Read the model definition and answer for the solid it produces. Units are mm, in the model's axes. A direction names the side the tool comes from. Coordinates: 2 decimals unless noted, no trailing zeros. Write each loop counter-clockwise with the first axis right and the second up, starting at its lowest first coordinate (ties: lowest second). Pieces come first, ordered by that corner, then holes. Notation, with made-up numbers: (20, -12) - (52, -12) arc R9 cw to (52, -3) - close; hole circle Ø6 at (-20.5, 27.5). An arc over 180 degrees is marked (long way). Return JSON: item names as keys, results as strings.
```python
from build123d import *

# Parameters (mm, degrees)
SKETCH1_R           = 15
BOSS_EXTRUDE1_DEPTH = 23.5
SKETCH2_R           = 1.65
CUT_EXTRUDE1_DEPTH  = 10


with BuildPart() as part:
    # Sketch1 → Boss-Extrude1 (new, symmetric)
    with BuildSketch(Plane.XY):
        Circle(SKETCH1_R)
    extrude(amount=BOSS_EXTRUDE1_DEPTH, both=True)

    # Sketch2 → Cut-Extrude1 (cut)
    with BuildSketch(Plane(origin=(0, 0, -23.5), x_dir=(-1, 0, 0), z_dir=(0, 0, -1))):
        with Locations((8, 8)):
            Circle(SKETCH2_R)
        with Locations((8, -8)):
            Circle(SKETCH2_R)
        with Locations((-8, -8)):
            Circle(SKETCH2_R)
        with Locations((-8, 8)):
            Circle(SKETCH2_R)
    extrude(amount=-CUT_EXTRUDE1_DEPTH, mode=Mode.SUBTRACT)


solid = part.part
```
(1) Which of the six approach directions +Z, -Z, +X, -X, +Y, -Y give full straight-line access (tool end or side, diameter ignored) to faces 4 (the face through (0, 0, -23.5)), 5 (the face through (9.65, -7.93, -18.57))?
Answer:
{"face 4": "-Z, +X, -X, +Y, -Y", "face 5": "-Z"}
(2) Determine the mould class of faces 1 (the face through (-14.985, 0.66, 0.329)), 2 (the face through (0, 0, 23.5)), 3 (the face through (-6.784, 9.115, -18.57)) for opening direction Y: +Y half, -Y half, draft (parallel to the pull), parting line (faces both ways), or undercut.
Answer:
{"face 1": "parting line", "face 2": "draft", "face 3": "undercut"}
(3) Straight lines are drawn through the part: line 1 (Y direction, x = 8, z = -19); line 2 (Z direction, x = -8.5, y = 9.5); line 3 (X direction, y = 1.25, z = 15.5). For each, find the intervals that lie inside material, in ascending order. Write a range as from..to.
Answer:
{"line 1": "-12.69..-9.65, -6.35..6.35, 9.65..12.69", "line 2": "-13.5..23.5", "line 3": "-14.95..14.95"}
(4) A cutting plane is placed at D-D (y = -4). Determine the outline of the cut face in (x, z), and give its area (3 significant figures).
Answer:
{"outline": "(-14.46, -23.5) - (14.46, -23.5) - (14.46, 23.5) - (-14.46, 23.5) - close", "area": "1,360 mm²"}
(5) A cutting plane is placed at B-B (y = 8). Determine the outline of the cut face in (x, z), and give its area (3 significant figures).
Answer:
{"outline": "(-12.69, -23.5) - (-9.65, -23.5) - (-9.65, -13.5) - (-6.35, -13.5) - (-6.35, -23.5) - (6.35, -23.5) - (6.35, -13.5) - (9.65, -13.5) - (9.65, -23.5) - (12.69, -23.5) - (12.69, 23.5) - (-12.69, 23.5) - close", "area": "1,130 mm²"}
(6) A cutting plane is placed at C-C (z = -8). Determine the outline of the cut face in (x, y), and give its area (3 significant figures).
Answer:
{"outline": "circle Ø30 at (0, 0)", "area": "707 mm²"}
(7) A cutting plane is placed at A-A (x = -9). Determine the outline of the cut face in (y, z), and give its area (3 significant figures).
Answer:
{"outline": "(-12, -23.5) - (-9.31, -23.5) - (-9.31, -13.5) - (-6.69, -13.5) - (-6.69, -23.5) - (6.69, -23.5) - (6.69, -13.5) - (9.31, -13.5) - (9.31, -23.5) - (12, -23.5) - (12, 23.5) - (-12, 23.5) - close", "area": "1,080 mm²"}
(8) Flat-ended cylindrical pins translate along their axes: P1, Ø1.5, axis at x = -8.5, z = 17, coming from the -Y side; P2, Ø1.5, axis at x = -3.5, z = 13.5, coming from the -Y side; P3, Ø1, axis at x = -8, z = 7, coming from the +Y side. Find the tip coordinate at first contact, or state that the pin passes through.
Answer:
{"P1": "y = -12.84", "P2": "y = -14.75", "P3": "y = 12.99"}
